from build123d import *

# Parameters (mm, degrees)
SKETCH1_W              = 266.7
SKETCH1_H              = 209.55
BOSS_EXTRUDE1_DEPTH    = 6.35
M3_CLEARANCE_HOLE1_D   = 3.6
SKETCH4_W              = 223.52
SKETCH4_H              = 153.67
CUT_EXTRUDE1_DEPTH     = 170.706645789
F_10_CLEARANCE_HOLE1_D = 5.6134
FILLET1_R              = 6.35


with BuildPart() as part:
    # Sketch1 → Boss-Extrude1 (new body)
    with BuildSketch(Plane(origin=(0, 0, 0), x_dir=(1, 0, 0), z_dir=(0, 1, 0))):
        Rectangle(SKETCH1_W, SKETCH1_H)
    extrude(amount=BOSS_EXTRUDE1_DEPTH)

    # M3 Clearance Hole1 (through all)
    with Locations(Plane(origin=(0, 6.35, 0), x_dir=(1, 0, 0), z_dir=(0, 1, 0))):
        with Locations((121.0056, -92.4306), (-121.0056, -92.4306), (-121.0056, 92.4306), (121.0056, 92.4306)):
            Hole(M3_CLEARANCE_HOLE1_D / 2)

    # Sketch4 → Cut-Extrude1 (cut, through all)
    with BuildSketch(Plane(origin=(0, 6.35, 0), x_dir=(1, 0, 0), z_dir=(0, 1, 0))):
        Rectangle(SKETCH4_W, SKETCH4_H)
    extrude(amount=-CUT_EXTRUDE1_DEPTH, mode=Mode.SUBTRACT)

    # #10 Clearance Hole1 (through all)
    with Locations(Plane(origin=(0, 6.35, 0), x_dir=(1, 0, 0), z_dir=(0, 1, 0))):
        with Locations((-61.9125, -87.1474), (-43.65625, -87.1474), (-25.4, -87.1474), (25.4, -87.1474), (43.65625, -87.1474), (61.9125, -87.1474)):
            Hole(F_10_CLEARANCE_HOLE1_D / 2)

    # Fillet1
    fillet1_edges = [part.edges().sort_by_distance(p)[0] for p in [
        (-111.76, 3.175, 76.835),
        (-111.76, 3.175, -76.835),
        (111.76, 3.175, -76.835),
        (111.76, 3.175, 76.835),
    ]]
    fillet(fillet1_edges, radius=FILLET1_R)


solid = part.part
Work out the finished part from the listing and answer in its coordinate system (mm). A direction names the side the tool comes from. Give positions to 0.01 mm unless a question says otherwise; leave off trailing zeros. Loops run counter-clockwise (first coordinate to the right, second up) from the corner with the lowest first, then second, coordinate; pieces in that order, holes last. Notation, with made-up numbers: (88, 78) -> (123, 78) arc R25 ccw to (123, 112) -> close; hole circle Ø1 at (28, 13.5). An arc over 180 degrees is marked (long way). Use a Markdown table: item, result. Add a question column.
1. Section A-A on z = -66 is taken. Determine the outline of the cut face in (x, y), and give its area (3 significant figures).
2. For faces 4 (the flat face through (-133.35, 3, 1)), 5 (the cylindrical face through (109.949, 3.131, -74.925)), determine the directions among +Z, -Z, +X, -X, +Y, -Y from which every point of the face is accessible in a straight line to the end or side of a thin tool.
3. Find the intervals of material crossed by probe 1 along Z at (x, y) = (-32.5, 5) (3 decimals); probe 2 along X at (y, z) = (1, 56); probe 3 along Z at (x, y) = (25.5, 4.5) (3 decimals), in increasing order.
4. Determine the mould class of faces 1 (the flat face through (111.76, 3, 1)), 2 (the flat face through (-2, 0, -95)), 3 (the flat face through (-2, 3, 104.775)) for opening direction Z: released by +Z, released by -Z, zero draft, split by the parting line, or undercut.
5. Section D-D on y = 3.5 is taken. State how many separate pieces and enclosed holes the cut face has, and give its area (3 significant figures).
6. Section C-C on x = -94.5 is taken. Determine the outline of the cut face in (y, z) (3 decimals).
7. Section B-B on x = 25.4 is taken. Determine the outline of the cut face in (y, z) (3 decimals).
8. Flat-ended cylindrical pins translate along their axes: pin 1 Ø3.5 at (x, z) = (-43.66, 87.15) entering from +Y; pin 2 Ø6 at (x, z) = (-121.01, -92.43) entering from -Y. Find the tip coordinate at first contact, or state that the pin passes through.
Results below:
| question | item | result |
|---|---|---|
| 1 | outline | (-133.35, 0) -> (-111.76, 0) -> (-111.76, 6.35) -> (-133.35, 6.35) -> close; (111.76, 0) -> (133.35, 0) -> (133.35, 6.35) -> (111.76, 6.35) -> close |
| 1 | area | 274 mm^2 |
| 2 | face 4 | +Z, -Z, -X, +Y, -Y |
| 2 | face 5 | +Y, -Y |
| 3 | probe 1 | z = -104.775 to -76.835, 76.835 to 104.775 |
| 3 | probe 2 | x = -133.35 to -111.76, 111.76 to 133.35 |
| 3 | probe 3 | z = -104.775 to -76.835, 76.835 to 84.342, 89.952 to 104.775 |
| 4 | face 1 | undercut |
| 4 | face 2 | zero draft |
| 4 | face 3 | released by +Z |
| 5 | separate pieces | 1 |
| 5 | enclosed holes | 11 |
| 5 | area | 21,400 mm^2 |
| 6 | outline | (0, -104.775) -> (6.35, -104.775) -> (6.35, -76.835) -> (0, -76.835) -> close; (0, 76.835) -> (6.35, 76.835) -> (6.35, 104.775) -> (0, 104.775) -> close |
| 7 | outline | (0, -104.775) -> (6.35, -104.775) -> (6.35, -76.835) -> (0, -76.835) -> close; (0, 76.835) -> (6.35, 76.835) -> (6.35, 84.341) -> (0, 84.341) -> close; (0, 89.954) -> (6.35, 89.954) -> (6.35, 104.775) -> (0, 104.775) -> close |
| 8 | pin 1 | passes through |
| 8 | pin 2 | stops at y = 0 |
